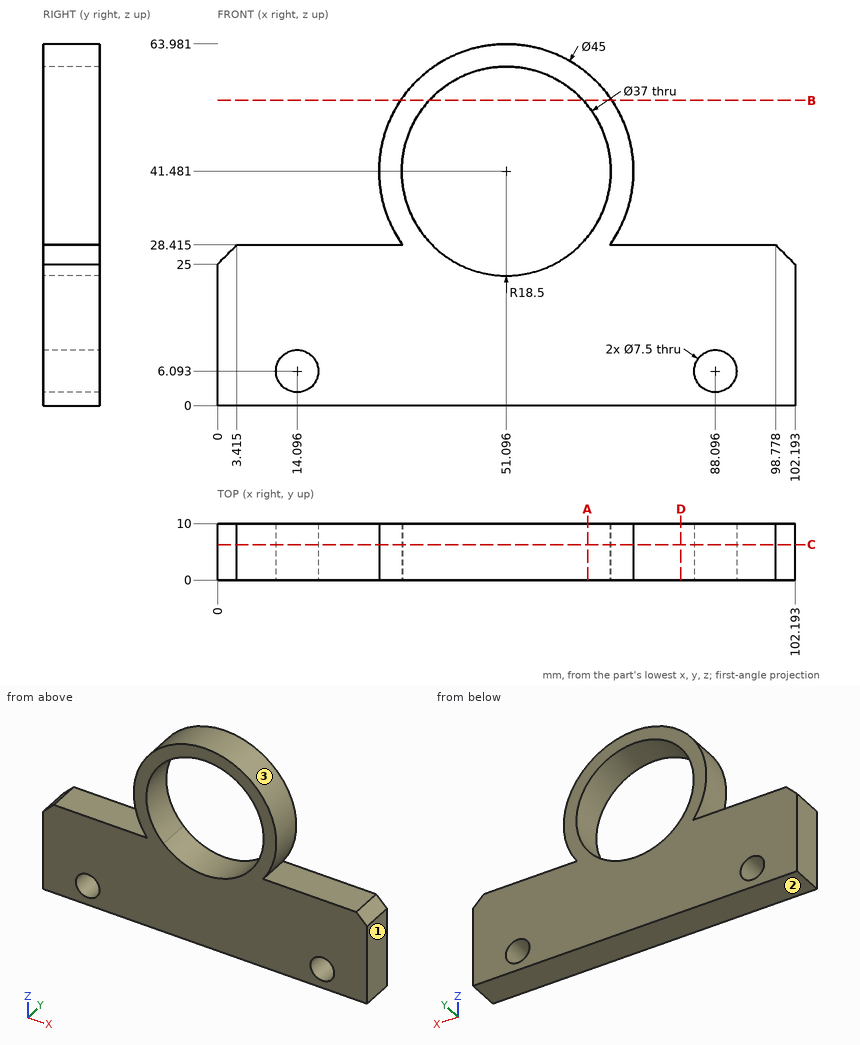
For this review, use the dimensioned drawing (mm, ordinates from the lowest corner) and the shaded views. Round coordinates to 2 decimals unless told otherwise and drop trailing zeros. Write each loop counter-clockwise with the first axis right and the second up, starting at its lowest first coordinate (ties: lowest second). Pieces come first, ordered by that corner, then holes. Notation, with made-up numbers: (4, 40.5) -> (39, 40.5) arc R34 ccw to (39, 74.5) -> close; hole circle Ø10 at (-2.5, 40). An arc over 180 degrees is marked (long way). Answer in a Markdown table with one row per item.
Q1. Draft analysis for pull direction Z (two halves, no side actions). For the marked faces 1, 2 and 3, state which applies: +Z half, -Z half, draft (parallel to the pull), parting line (faces both ways), or undercut.
The answers:
| item | result |
|---|---|
| face 1 | draft |
| face 2 | -Z half |
| face 3 | undercut |
Q2. Clearance check with flat-ended pins moving along their axes: pin 1 Ø10 at (x, z) = (87, 34) entering from -Y; pin 2 Ø1 at (y, z) = (7.5, 33) entering from +X; pin 3 Ø3 at (x, y) = (12, 3.5) entering from +Z (1 decimal); pin 4 Ø5 at (x, z) = (45.5, 57) entering from -Y. State where each tip first meets the part, or that it passes through.
The answers:
| item | result |
|---|---|
| pin 1 | through |
| pin 2 | x = 72.13 |
| pin 3 | z = 28.4 |
| pin 4 | y = 0 |
Q3. Take a section at C-C, the plane y = 6.25. Count the separate pieces of the cut face and the enclosed holes in it, then the cut area to 3 significant figures.
The answers:
| item | result |
|---|---|
| separate pieces | 1 |
| enclosed holes | 3 |
| area | 3,080 mm² |
Q4. Take a section at D-D, the plane x = 82. State the section outline as (y, z) points (1 decimal), then the cut area to 3 significant figures.
The answers:
| item | result |
|---|---|
| outline | (0, 0) -> (10, 0) -> (10, 28.4) -> (0, 28.4) -> close |
| area | 284 mm² |
Q5. Take a section at B-B, the plane z = 54. State the section outline as (x, y) points.
The answers:
| item | result |
|---|---|
| outline | (32.4, 0) -> (37.48, 0) -> (37.48, 10) -> (32.4, 10) -> close; (64.72, 0) -> (69.79, 0) -> (69.79, 10) -> (64.72, 10) -> close |
Q6. Take a section at A-A, the plane x = 65.5. State the section outline as (y, z) points.
The answers:
| item | result |
|---|---|
| outline | (0, 0) -> (10, 0) -> (10, 29.87) -> (0, 29.87) -> close; (0, 53.09) -> (10, 53.09) -> (10, 58.77) -> (0, 58.77) -> close |
Q7. To check wall thickness, follow L1, parallel to X at y = 1.25, z = 6.5 (1 decimal); L2, parallel to Z at x = 51.5, y = 4.5 (1 decimal); L3, parallel to X at y = 5.75, z = 7 (1 decimal). State the ranges of each line that lie inside material, in increasing order. Write a range as [from, to].
The answers:
| item | result |
|---|---|
| L1 | [0, 10.4], [17.8, 84.4], [91.8, 102.2] |
| L2 | [0, 23], [60, 64] |
| L3 | [0, 10.5], [17.7, 84.5], [91.7, 102.2] |
